CAD build for the part. Positions are in the model's coordinates, mm. A direction names the side the tool comes from. Coordinates: 2 decimals unless noted, no trailing zeros. Order: outer loops, then holes, each group sorted by start corner. A loop starts at its lowest first (then second) coordinate and runs counter-clockwise, first axis right, second up.
from build123d import *

# Parameters (mm, degrees)
SKETCH1_W           = 76.2
SKETCH1_H           = 25.4
BOSS_EXTRUDE1_DEPTH = 12.7
SKETCH2_R           = 5.08
CUT_EXTRUDE1_DEPTH  = 43.121134838
SKETCH3_R           = 1.905
CUT_EXTRUDE2_DEPTH  = 43.121134838
SKETCH4_W           = 40.64
SKETCH4_H           = 20.32
SKETCH4_W_2         = 5.703951
SKETCH4_H_2         = 2.54
CUT_EXTRUDE3_DEPTH  = 8.599932
SKETCH5_R           = 6.985
CUT_EXTRUDE4_DEPTH  = 1.999996
SKETCH9_R           = 6.35
BOSS_EXTRUDE3_DEPTH = 12.7
SKETCH7_R           = 3.175
CUT_EXTRUDE5_DEPTH  = 12.7


with BuildPart() as part:
    # Sketch1 → Boss-Extrude1 (new body)
    with BuildSketch(Plane.XY):
        Rectangle(SKETCH1_W, SKETCH1_H)
    extrude(amount=BOSS_EXTRUDE1_DEPTH)

    # Sketch2 → Cut-Extrude1 (cut, through all)
    with BuildSketch(Plane.XY.offset(12.7)):
        with Locations((20.32, 0)):
            Circle(SKETCH2_R)
        with Locations(Location((-20.32, 0, 0), (0, 0, 180))):
            Circle(SKETCH2_R)
    extrude(amount=-CUT_EXTRUDE1_DEPTH, mode=Mode.SUBTRACT)

    # Sketch3 → Cut-Extrude2 (cut, through all)
    with BuildSketch(Plane.XY.offset(12.7)):
        with Locations((34.820098, 4.99999)):
            Circle(SKETCH3_R)
        with Locations((-14.179804, 4.99999)):
            Circle(SKETCH3_R)
        with Locations(Location((34.820098, -4.99999, 0), (0, 0, 180))):
            Circle(SKETCH3_R)
        with Locations(Location((-14.179804, -4.99999, 0), (0, 0, 180))):
            Circle(SKETCH3_R)
    extrude(amount=-CUT_EXTRUDE2_DEPTH, mode=Mode.SUBTRACT)

    # Sketch4 → Cut-Extrude3 (cut)
    with BuildSketch(Plane(origin=(0, 0, 0), x_dir=(-1, 0, 0), z_dir=(0, 0, -1))):
        with Locations((-10.320147, 0)):
            Rectangle(SKETCH4_W, SKETCH4_H)
        with Locations((-33.4921225, 0)):
            Rectangle(SKETCH4_W_2, SKETCH4_H_2)
        with Locations((12.8518285, 0)):
            Rectangle(SKETCH4_W_2, SKETCH4_H_2)
    extrude(amount=-CUT_EXTRUDE3_DEPTH, mode=Mode.SUBTRACT)

    # Sketch5 → Cut-Extrude4 (cut)
    with BuildSketch(Plane(origin=(0, 0, 8.599932), x_dir=(-1, 0, 0), z_dir=(0, 0, -1))):
        with Locations((-20.32, 0)):
            Circle(SKETCH5_R)
    extrude(amount=-CUT_EXTRUDE4_DEPTH, mode=Mode.SUBTRACT)

    # Sketch9 → Boss-Extrude3 (add)
    with BuildSketch(Plane.XZ.offset(12.7)):
        with Locations(Location((0, 6.35, 0), (0, 0, 270))):
            Circle(SKETCH9_R)
    extrude(amount=BOSS_EXTRUDE3_DEPTH)

    # Sketch7 → Cut-Extrude5 (cut)
    with BuildSketch(Plane.XZ.offset(25.4)):
        with Locations(Location((0, 6.35, 0), (0, 0, 270))):
            Circle(SKETCH7_R)
    extrude(amount=-CUT_EXTRUDE5_DEPTH, mode=Mode.SUBTRACT)


solid = part.part
1) Two-plate mould, pull along X, no slides. Class faces 1 (the cylindrical face through (-16.083, 5.084, 6.439)), 2 (the cylindrical face through (1.907, -18.961, 0.293)), 3 (the flat face through (23, -12.7, 6)): released by +X, released by -X, zero draft, split by the parting line, or undercut.
2) Slice it at B-B (y = 0). List the corners of the cut face in (x, z) (3 decimals), plus the area to 3 significant figures.
3) Slice it at C-C (z = 2.25). List the corners of the cut face in (x, y) (3 decimals).
4) Which spindle directions (+Z, -Z, +X, -X, +Y, -Y) get a long thin tool onto all of the face, cutting with end or side? Do faces 4 (the flat face through (0, -12.7, 6)), 5 (the flat face through (-13, 1.27, 4)), 6 (the cylindrical face through (-25.165, -1.526, 6.439)). Say none if no direction does.
5) Slice it at A-A (x = -20.32). List the corners of the cut face in (y, z), plus the area to 3 significant figures.
6) Drill centre lines: probe 1 along Y at (x, z) = (30, 3.25); probe 2 along X at (y, z) = (7, 6.5); probe 3 along Y at (x, z) = (-11.5, 4.5). Where is each one in solid material? Low to high.
7) Pin check, flat tips, straight feed: P1, Ø4, axis at x = 23.5, y = -2.5, coming from the -Z side; P2, Ø2, axis at x = 0.5, z = 7, coming from the -Y side; P3, Ø10, axis at x = 17, y = 2.5, coming from the -Z side. Stop position of each tip, or through.
8) Slice it at D-D (x = -7.5). List the corners of the cut face in (y, z), plus the area to 3 significant figures.
Worked out:
1. face 1: undercut
1. face 2: split by the parting line
1. face 3: zero draft
2. outline: (-38.1, 0) - (-25.4, 0) - (-25.4, 12.7) - (-38.1, 12.7) - close; (-15.24, 8.6) - (13.335, 8.6) - (13.335, 10.6) - (15.24, 10.6) - (15.24, 12.7) - (-15.24, 12.7) - close; (25.4, 10.6) - (27.305, 10.6) - (27.305, 8.6) - (36.344, 8.6) - (36.344, 0) - (38.1, 0) - (38.1, 12.7) - (25.4, 12.7) - close
2. area: 346 mm2
3. outline: (-38.1, -12.7) - (-4.849, -12.7) - (-4.849, -25.4) - (4.849, -25.4) - (4.849, -12.7) - (38.1, -12.7) - (38.1, 12.7) - (-38.1, 12.7) - close; hole circle Ø3.81 at (-14.18, -5); hole circle Ø3.81 at (-14.18, 5); hole (-15.401, -1.27) - (-10, -1.27) - (-10, -10.16) - (30.64, -10.16) - (30.64, -1.27) - (36.344, -1.27) - (36.344, 1.27) - (30.64, 1.27) - (30.64, 10.16) - (-10, 10.16) - (-10, 1.27) - (-15.401, 1.27) arc R5.08 ccw (long way) to start; hole circle Ø3.81 at (34.82, -5); hole circle Ø3.81 at (34.82, 5)
4. face 4: -Y
4. face 5: -Z
4. face 6: +Z, -Z
5. outline: (-12.7, 0) - (-5.08, 0) - (-5.08, 12.7) - (-12.7, 12.7) - close; (5.08, 0) - (12.7, 0) - (12.7, 12.7) - (5.08, 12.7) - close
5. area: 194 mm2
6. probe 1: y = -12.7 to -10.16, 10.16 to 12.7
6. probe 2: x = -38.1 to -10, 30.64 to 38.1
6. probe 3: y = -12.7 to -1.27, 1.27 to 12.7
7. P1: stops at z = 10.6
7. P2: stops at y = -12.7
7. P3: stops at z = 8.6
8. outline: (-12.7, 0) - (-10.16, 0) - (-10.16, 8.6) - (10.16, 8.6) - (10.16, 0) - (12.7, 0) - (12.7, 12.7) - (-12.7, 12.7) - close
8. area: 148 mm2
